from build123d import *

# Parameters (mm, degrees)
SKETCH1_R           = 4.7625
EXTRUDE1_DEPTH      = 17.78
EXTRUDE2_DEPTH      = 20.01292225
EXTRUDE2_DEPTH_BACK = 20.01292225


with BuildPart() as part:
    # Sketch1 → Extrude1 (new body)
    with BuildSketch(Plane.XY):
        Circle(SKETCH1_R)
    extrude(amount=EXTRUDE1_DEPTH)

    # Sketch2 → Extrude2 (cut, two sides: drawn at the far end of the back side and taken through both)
    with BuildSketch(Plane(origin=(0, 0, 0), x_dir=(1, 0, 0), z_dir=(0, 1, 0)).offset(-EXTRUDE2_DEPTH_BACK)):
        Polygon((0, 0), (4.7625, -4.7625), (4.7625, 1.90519665), (-4.7625, 1.90519665), (-4.7625, -4.7625), align=None)
    extrude(amount=EXTRUDE2_DEPTH + EXTRUDE2_DEPTH_BACK, mode=Mode.SUBTRACT)

    # Sketch5 → 1/8 (0.125) Diameter Hole1 (revolve, cut)
    with BuildSketch(Plane(origin=(0, 0, 9.8298), x_dir=(0, 0, 1), z_dir=(0, 1, 0))):
        Polygon((0, 0), (0, 16.955866233), (1.5875, 16.002), (1.5875, 0), align=None)
    revolve(axis=Axis((-6.35, 0, 9.8298), (1, 0, 0)), mode=Mode.SUBTRACT)


solid = part.part
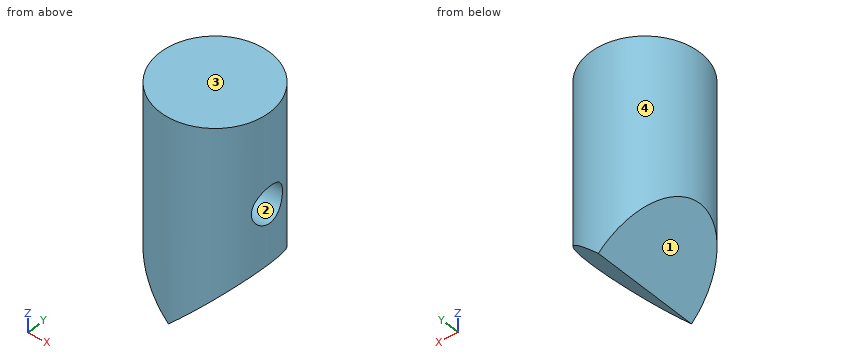
Source: CAD feature listing. Evaluate the final solid. Frame: model axes, mm. Face numbers are marked on the shaded views. Give positions to 0.01 mm unless a question says otherwise; leave off trailing zeros. Order: outer loops, then holes, each group sorted by start corner. A loop starts at its lowest first (then second) coordinate and runs counter-clockwise, first axis right, second up. Notation, with made-up numbers: (3, -2) -> (28, -2) arc R30 ccw to (28, 22) -> close; hole circle Ø10 at (15.5, 5). An arc over 180 degrees is marked (long way). Use a Markdown table: item, result.
1) Section query A-A, the plane y = 0. Return the cut outline in (x, z).
Answer list:
| item | result |
|---|---|
| outline | (-4.76, 4.76) -> (0, 0) -> (4.76, 4.76) -> (4.76, 8.24) -> (0, 8.24) -> (0, 11.42) -> (4.76, 11.42) -> (4.76, 17.78) -> (-4.76, 17.78) -> close |
2) Contact query for flat-ended pins moving along their axis: P1, Ø3, axis at y = -1.5, z = 5, coming from the +X side; P2, Ø3, axis at x = 3, z = 9.5, coming from the +Y side; P3, Ø1, axis at x = -3, z = 7, coming from the +Y side; P4, Ø2, axis at x = -2, z = 4, coming from the +Y side. Output: stop coordinate, or through.
Answer list:
| item | result |
|---|---|
| P1 | x = 4.76 |
| P2 | y = 4.52 |
| P3 | y = 4.05 |
| P4 | y = 4.66 |
3) Section query B-B, the plane x = 4. Return the cut outline in (y, z) (1 decimal).
Answer list:
| item | result |
|---|---|
| outline | (-2.6, 4) -> (2.6, 4) -> (2.6, 17.8) -> (-2.6, 17.8) -> close; hole circle Ø3.2 at (0, 9.8) |
4) Section query C-C, the plane z = 13.5. Return the cut outline in (x, y) (1 decimal), then the cut area to 3 significant figures.
Answer list:
| item | result |
|---|---|
| outline | circle Ø9.5 at (0, 0) |
| area | 71.3 mm² |
5) Section query D-D, the plane x = -1. Return the cut outline in (y, z), then the cut area to 3 significant figures.
Answer list:
| item | result |
|---|---|
| outline | (-4.66, 1) -> (4.66, 1) -> (4.66, 17.78) -> (-4.66, 17.78) -> close |
| area | 156 mm² |
6) Ray query, line 1 along Z through (x, y) = (2.95, 0); line 2 along X through (y, z) = (-1, 8.25). Return the intervals inside material, ascending. Write a range as [from, to].
Answer list:
| item | result |
|---|---|
| line 1 | [2.95, 8.24], [11.42, 17.78] |
| line 2 | [-4.66, 4.66] |
7) Mould query, pull axis Z, two halves, no side actions, for the marked faces 1, 2, 3 and 4. Classes: +Z half, -Z half, draft (parallel to the pull), parting line (faces both ways), or undercut.
Answer list:
| item | result |
|---|---|
| face 1 | -Z half |
| face 2 | undercut |
| face 3 | +Z half |
| face 4 | draft |
